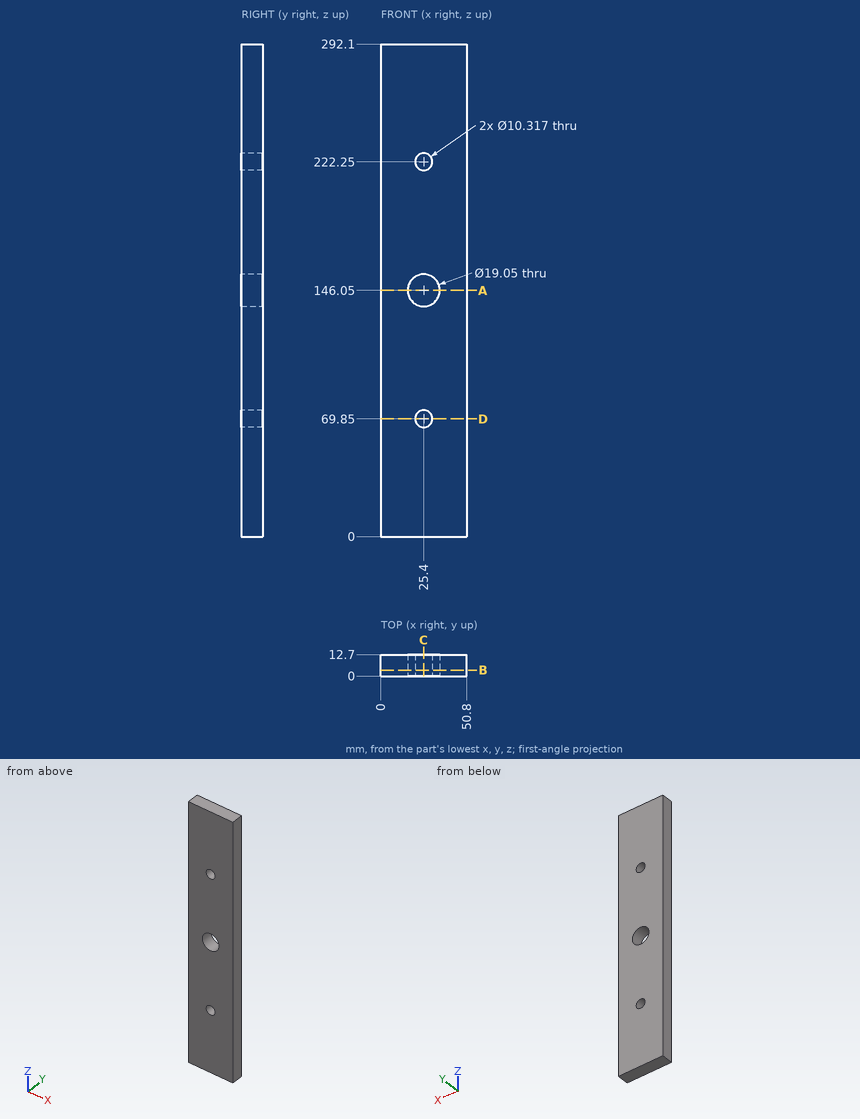
Check sheet for the drawn part. Datum: minimum x, y, z corner. Units: mm. Coordinates: 2 decimals unless noted, no trailing zeros. Loops run counter-clockwise (first coordinate to the right, second up) from the corner with the lowest first, then second, coordinate; pieces in that order, holes last. Notation, with made-up numbers: (53.5, 42) -> (79.5, 42) arc R25 cw to (79.5, 57) -> close; hole circle Ø1 at (37, 61.5). An arc over 180 degrees is marked (long way). Answer as a JSON object with one key per item and string values. Group by question number.
Item 1: Sectioned sample at B-B on y = 3.5. State how many separate pieces and enclosed holes the cut face has, plus the area to 3 significant figures.
Item 2: Sectioned sample at D-D on z = 69.85. Record the boundary of the cut face in (x, y), plus the area to 3 significant figures.
Item 3: Scan lines: probe 1 along X at (y, z) = (2.75, 146.05) (1 decimal); probe 2 along Z at (x, y) = (23.5, 7.5) (1 decimal). Record each from-to range of solid material in increasing order.
Item 4: Sectioned sample at C-C on x = 25.4. Record the boundary of the cut face in (y, z) (1 decimal), plus the area to 3 significant figures.
Item 5: Sectioned sample at A-A on z = 146.05. Record the boundary of the cut face in (x, y) (1 decimal).
Item 6: Depth check by flat-ended pin: pin 1 (11.5 mm diameter, centred on x = 25.4, z = 146.05, fed in from -Y). Enter the tip coordinate at first touch or a pass-through.
Evaluation:
{
 "1": {"separate pieces": "1", "enclosed holes": "3", "area": "14,400 mm²"},
 "2": {"outline": "(0, 0) -> (20.24, 0) -> (20.24, 12.7) -> (0, 12.7) -> close; (30.56, 0) -> (50.8, 0) -> (50.8, 12.7) -> (30.56, 12.7) -> close", "area": "514 mm²"},
 "3": {"probe 1": "x = 0 to 15.9, 34.9 to 50.8", "probe 2": "z = 0 to 65.1, 74.6 to 136.7, 155.4 to 217.5, 227 to 292.1"},
 "4": {"outline": "(0, 0) -> (12.7, 0) -> (12.7, 64.7) -> (0, 64.7) -> close; (0, 75) -> (12.7, 75) -> (12.7, 136.5) -> (0, 136.5) -> close; (0, 155.6) -> (12.7, 155.6) -> (12.7, 217.1) -> (0, 217.1) -> close; (0, 227.4) -> (12.7, 227.4) -> (12.7, 292.1) -> (0, 292.1) -> close", "area": "3,210 mm²"},
 "5": {"outline": "(0, 0) -> (15.9, 0) -> (15.9, 12.7) -> (0, 12.7) -> close; (34.9, 0) -> (50.8, 0) -> (50.8, 12.7) -> (34.9, 12.7) -> close"},
 "6": {"pin 1": "passes through"}
}
